Here's how the part is built. I have some questions about the finished solid (model axes, mm). Give positions to 0.01 mm unless a question says otherwise; leave off trailing zeros. Write each loop counter-clockwise with the first axis right and the second up, starting at its lowest first coordinate (ties: lowest second). Pieces come first, ordered by that corner, then holes. Notation, with made-up numbers: (1, -24) -> (53, -24) arc R17 cw to (53, -15) -> close; hole circle Ø8 at (-2.5, -2). An arc over 180 degrees is marked (long way). Put each result on its own line as item: value. Start each with the question number.
from build123d import *

# Parameters (mm, degrees)
F1_DEPTH = 17.526
F0_W     = 304.8
F0_H     = 20.32
F2_DEPTH = 8.255
F0_H_2   = 297.18
F3_DEPTH = 17.526


with BuildPart() as f1:
    # F0 (on Front) → F1 (new body)
    with BuildSketch(Plane.XZ):
        with BuildLine():
            Line((8.833553, 146.481255), (-92.766447, 146.481255))
            Line((-92.766447, 146.481255), (-92.766447, -450.418745))
            Line((-92.766447, -450.418745), (212.033553, -450.418745))
            ThreePointArc((212.033553, -450.418745), (61.279772, -195.656633), (8.833553, 95.684799))
            Line((8.833553, 95.684799), (8.833553, 146.481255))
        make_face()
    extrude(amount=F1_DEPTH)

    # F0 (on Front) → F2 (join)
    with BuildSketch(Plane.XZ):
        with Locations((59.633553, -460.578745)):
            Rectangle(F0_W, F0_H)
    extrude(amount=F2_DEPTH)

    # F0 (on Front) → F3 (join)
    with BuildSketch(Plane.XZ):
        with Locations((59.633553, -619.328745)):
            Rectangle(F0_W, F0_H_2)
    extrude(amount=F3_DEPTH)


solid = f1.part
1) I want a section at D-D, the plane x = 73. Write out the boundary of the cut face in (y, z) (3 decimals), and give its area (3 significant figures).
2) I want a section at C-C, the plane z = -116. Write out the boundary of the cut face in (x, y), and give its area (3 significant figures).
3) I'm going to push a flat-ended pin straight in: pin 1 Ø10 at (x, z) = (7, -456.5) entering from -Y (3 decimals). Where does the tip first touch, or does it pass through?
4) I want a section at A-A, the plane y = -13.5. Write out the boundary of the cut face in (x, z).
5) Thinking about a two-plate mould opening in Z: for faces 1 (the flat face through (57, -8.255, -460)), 2 (the cylindrical face through (62.742, -8.64, -199.558)), 3 (the flat face through (8.834, -9, 121)), which applies, released by +Z, released by -Z, zero draft, split by the parting line, or undercut?
6) I want a section at B-B, the plane x = 120.5. Write out the boundary of the cut face in (y, z) (3 decimals).
7) I need wall thicknesses on probe 1 along Z at (x, y) = (-31, -12); probe 2 along Y at (x, z) = (102, -450.5) (3 decimals); probe 3 along Z at (x, y) = (150.5, -8.75). Which ranges of each line are inside material? Lowest first, please.
Established:
1. outline: (-17.526, -767.919) -> (0, -767.919) -> (0, -225.401) -> (-17.526, -225.401) -> (-17.526, -450.419) -> (-8.255, -450.419) -> (-8.255, -470.739) -> (-17.526, -470.739) -> close
1. area: 9,320 mm2
2. outline: (-92.77, -17.53) -> (36.1, -17.53) -> (36.1, 0) -> (-92.77, 0) -> close
2. area: 2,260 mm2
3. pin 1: stops at y = -8.255
4. outline: (-92.77, -767.92) -> (212.03, -767.92) -> (212.03, -470.74) -> (-92.77, -470.74) -> close; (-92.77, -450.42) -> (212.03, -450.42) arc R835.43 cw to (8.83, 95.68) -> (8.83, 146.48) -> (-92.77, 146.48) -> close
5. face 1: undercut
5. face 2: released by +Z
5. face 3: zero draft
6. outline: (-17.526, -767.919) -> (0, -767.919) -> (0, -321.58) -> (-17.526, -321.58) -> (-17.526, -450.419) -> (-8.255, -450.419) -> (-8.255, -470.739) -> (-17.526, -470.739) -> close
7. probe 1: z = -767.92 to -470.74, -450.42 to 146.48
7. probe 2: y = -8.255 to 0
7. probe 3: z = -767.92 to -470.74, -450.42 to -369.76
